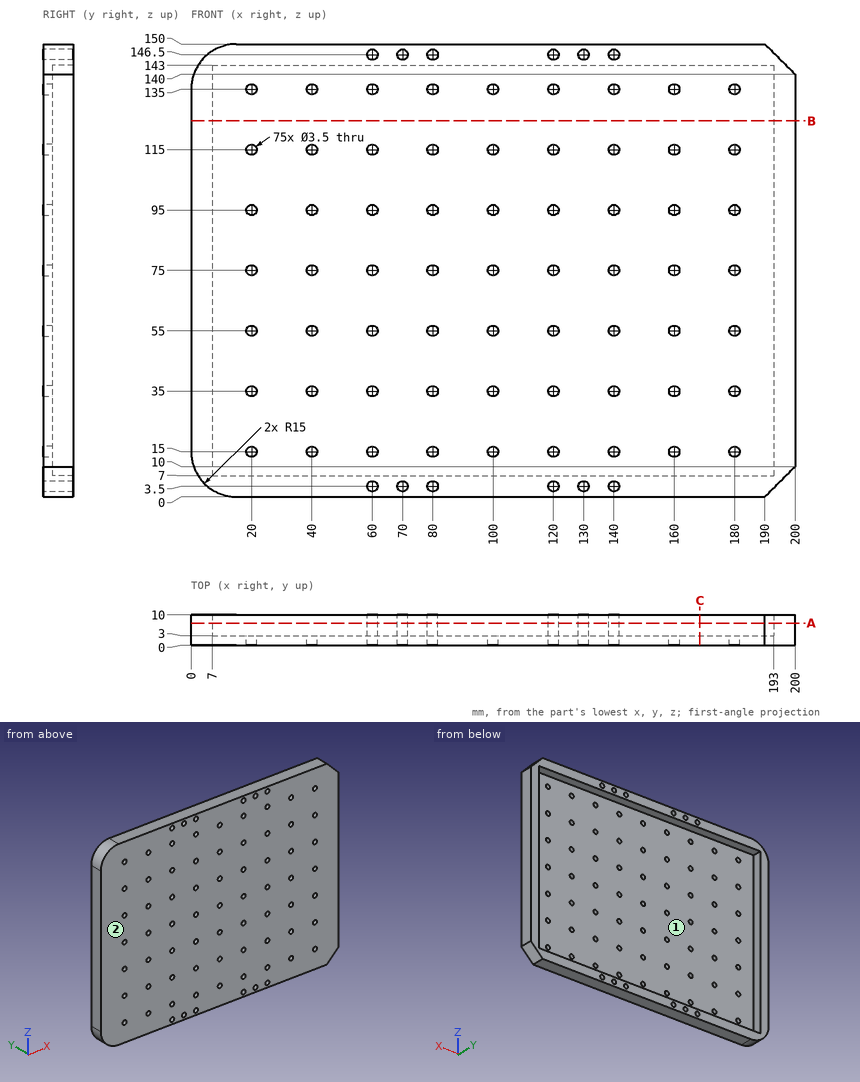
Verification items for this drawing (mm, ordinates from the low corner). Coordinates: 2 decimals unless noted, no trailing zeros. Order: outer loops, then holes, each group sorted by start corner. A loop starts at its lowest first (then second) coordinate and runs counter-clockwise, first axis right, second up. Notation, with made-up numbers: (87.5, -17) - (91.5, -17) arc R22 ccw to (91.5, 1) - close; hole circle Ø1 at (22, 26.25). An arc over 180 degrees is marked (long way). Answer as a JSON object with one key per item and string values. Group by question number.
Item 1: Scan lines: probe 1 along Z at (x, y) = (130, 5); probe 2 along X at (y, z) = (9.5, 114.5); probe 3 along Z at (x, y) = (41.5, 8). Record each from-to range of solid material in increasing order.
Item 2: Sectioned sample at C-C, the plane x = 168.5. Record the cut outline in (y, z), and give its area (3 significant figures).
Item 3: Draft check along X on the marked faces 1 and 2. Enter one of: +X half, -X half, draft (parallel to the pull), parting line (faces both ways), or undercut.
Item 4: Sectioned sample at A-A, the plane y = 7.25. Give the number of separate pieces and of enclosed holes in the cut face, and give its area (3 significant figures).
Item 5: Depth check by flat-ended pin: pin 1 Ø5.5 at (x, z) = (180, 135) entering from +Y. Enter the tip coordinate at first touch or a pass-through.
Item 6: Sectioned sample at B-B, the plane z = 124.5. Record the cut outline in (x, y), and give its area (3 significant figures).
Resolved:
{
 "1": {"probe 1": "0 to 1.75, 5.25 to 7, 143 to 144.75, 148.25 to 150", "probe 2": "0 to 7, 193 to 200", "probe 3": "0 to 7, 143 to 150"},
 "2": {"outline": "(0, 0) - (10, 0) - (10, 7) - (3, 7) - (3, 143) - (10, 143) - (10, 150) - (0, 150) - close", "area": "548 mm^2"},
 "3": {"face 1": "undercut", "face 2": "draft"},
 "4": {"separate pieces": "1", "enclosed holes": "13", "area": "4,390 mm^2"},
 "5": {"pin 1": "y = 3"},
 "6": {"outline": "(0, 0) - (200, 0) - (200, 10) - (193, 10) - (193, 3) - (7, 3) - (7, 10) - (0, 10) - close", "area": "698 mm^2"}
}
